Check sheet for the modelled part. Datum: model origin and axes. Units: mm. Face numbers are marked on the shaded views. A direction names the side the tool comes from. Coordinates: 2 decimals unless noted, no trailing zeros. Write each loop counter-clockwise with the first axis right and the second up, starting at its lowest first coordinate (ties: lowest second). Pieces come first, ordered by that corner, then holes. Notation, with made-up numbers: M 74,31 L 128,31 A14 ccw 128,39 Z; hole C 19,16.5 d6. An arc over 180 degrees is marked long. Answer as CSV lines item,"result". Start each with the question number.
Q1. Sectioned sample at B-B, the plane x = 25. Record the cut outline in (y, z).
Q2. Thickness scan on line 1 along X through (y, z) = (-9.5, 0.25); line 2 along Z through (x, y) = (25, -3.75); line 3 along X through (y, z) = (-7.5, -2). Record the ranges inside material, lowest first. Write a range as from..to.
Q3. Sectioned sample at A-A, the plane z = 0. Record the cut outline in (x, y), then the cut area to 3 significant figures.
Q4. Sectioned sample at D-D, the plane x = -9. Record the cut outline in (y, z).
Q5. Access from +Z, -Z, +X, -X, +Y, -Y to the whole of each face (thin tool, end or side, straight path). Record for the marked faces 1, 2 and 3.
Q6. Sectioned sample at C-C, the plane y = -1.25. Record the cut outline in (x, z).
Q7. Depth check by flat-ended pin: pin 1 Ø8 at (x, z) = (10.5, 14.5) entering from +Y; pin 2 Ø2 at (x, y) = (4.5, -1) entering from +Z. Enter the tip coordinate at first touch or a pass-through.
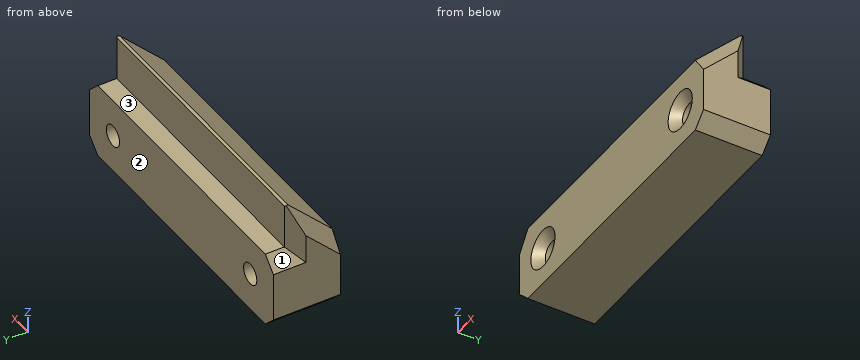
from build123d import *

# Parameters (mm, degrees)
F0_W     = 67
F0_H     = 17
F0_R     = 2.4
F0_H_2   = 10
F1_DEPTH = 15
F2_DEPTH = 4.25
F3_SIZE  = 2
F4_SIZE  = 10
F5_SIZE  = 3


with BuildPart() as f1:
    # F0 (on Front) → F1 (new body)
    with BuildSketch(Plane.XZ):
        Rectangle(F0_W, F0_H)
        with Locations((-25, 0)):
            Circle(F0_R, mode=Mode.SUBTRACT)
        with Locations((25, 0)):
            Circle(F0_R, mode=Mode.SUBTRACT)
        with Locations((0, 13.5)):
            Rectangle(F0_W, F0_H_2)
    extrude(amount=F1_DEPTH)

    # F0 (on Front) → F2 (cut)
    with BuildSketch(Plane.XZ):
        with Locations((0, 13.5)):
            Rectangle(F0_W, F0_H_2)
    extrude(amount=F2_DEPTH, mode=Mode.SUBTRACT)

    # F3
    f3_edges = [f1.edges().sort_by_distance(p)[0] for p in [
        (-27.4, -15, 0),
        (22.6, -15, 0),
    ]]
    chamfer(f3_edges, length=F3_SIZE)

    # F4
    f4_edges = [f1.edges().sort_by_distance(p)[0] for p in [
        (0, -15, 18.5),
    ]]
    chamfer(f4_edges, length=F4_SIZE)

    # F5 (call 1 of 6: OpenCascade refuses the feature's edges together)
    f5_edges = [f1.edges().sort_by_distance(p)[0] for p in [
        (-33.5, -10, 13.5),
    ]]
    chamfer(f5_edges, length=F5_SIZE)

    # F5#2 (call 2 of 6)
    f5_2_edges = [f1.edges().sort_by_distance(p)[0] for p in [
        (33.5, -10, 13.5),
    ]]
    chamfer(f5_2_edges, length=F5_SIZE)

    # F5#3 (call 3 of 6)
    f5_3_edges = [f1.edges().sort_by_distance(p)[0] for p in [
        (33.5, -7.5, -8.5),
    ]]
    chamfer(f5_3_edges, length=F5_SIZE)

    # F5#4 (call 4 of 6)
    f5_4_edges = [f1.edges().sort_by_distance(p)[0] for p in [
        (-33.5, -7.5, -8.5),
    ]]
    chamfer(f5_4_edges, length=F5_SIZE)

    # F5#5 (call 5 of 6)
    f5_5_edges = [f1.edges().sort_by_distance(p)[0] for p in [
        (33.5, -2.125, 8.5),
        (33.5, -4.25, 13.5),
    ]]
    chamfer(f5_5_edges, length=F5_SIZE)

    # F5#6 (call 6 of 6)
    f5_6_edges = [f1.edges().sort_by_distance(p)[0] for p in [
        (-33.5, -4.25, 13.5),
        (-33.5, -2.125, 8.5),
    ]]
    chamfer(f5_6_edges, length=F5_SIZE)


solid = f1.part
Output:
1,outline,"M -15,-8.5 L 0,-8.5 L 0,-2.4 L -13,-2.4 L -15,-4.4 Z; M -15,4.4 L -13,2.4 L 0,2.4 L 0,8.5 L -4.25,8.5 L -4.25,18.5 L -5,18.5 L -15,8.5 Z"
2,line 1,"x = -33.5..-27.39, -22.61..22.61, 27.39..33.5"
2,line 2,"z = -8.5..-2.4, 2.4..8.5"
2,line 3,"x = -33.5..-26.33, -23.67..23.67, 26.33..33.5"
3,outline,"M -33.5,-15 L -29.4,-15 L -27.4,-13 L -27.4,0 L -33.5,0 Z; M -22.6,-13 L -20.6,-15 L 20.6,-15 L 22.6,-13 L 22.6,0 L -22.6,0 Z; M 27.4,-13 L 29.4,-15 L 33.5,-15 L 33.5,0 L 27.4,0 Z"
3,area,"853 mm^2"
4,outline,"M -15,-8.5 L 0,-8.5 L 0,8.5 L -4.25,8.5 L -4.25,18.5 L -5,18.5 L -15,8.5 Z"
5,face 1,"+Z, -X, +Y"
5,face 2,"+Z, -Z, +X, -X, +Y"
5,face 3,"+Z, +X, -X, +Y"
6,outline,"M -33.5,-5.5 L -30.5,-8.5 L 30.5,-8.5 L 33.5,-5.5 L 33.5,5.5 L 30.5,8.5 L -30.5,8.5 L -33.5,5.5 Z; hole C -25,0 d4.8; hole C 25,0 d4.8"
7,pin 1,"stops at y = -4.25"
7,pin 2,"stops at z = 8.5"
